Can you work these out from the model? Positions are in its coordinate system, mm. Face numbers are marked on the shaded views. A direction names the side the tool comes from. Round coordinates to 2 decimals unless told otherwise and drop trailing zeros. Loops run counter-clockwise (first coordinate to the right, second up) from the corner with the lowest first, then second, coordinate; pieces in that order, holes last.
(1) I want a section at C-C on x = 223. Write out the boundary of the cut face in (y, z).
(2) I want a section at A-A on y = -32. Write out the boundary of the cut face in (x, z).
(3) Thinking about a two-plate mould opening in Y: for the marked faces 3 and 4, which applies, released by +Y, released by -Y, zero draft, split by the parting line, or undercut?
(4) Which directions (+Z, -Z, +X, -X, +Y, -Y) give clear straight access to the entire face, cutting with the end or side of a thin tool? Please do the marked faces 1 and 2.
(5) If I drill on line 1 along Y through (x, z) = (129, 12); line 2 along Z through (x, y) = (30, -19); line 3 along Z through (x, y) = (85, -36), over which ranges is the centre line in solid material (lowest first)?
(6) I want a section at B-B on z = 59. Write out the boundary of the cut face in (x, y), plus the area to 3 significant figures.
(7) Will these pins go through, and if not, where does the flat tip stop? pin 1 Ø5 at (y, z) = (-23, 15.5) entering from -X; pin 2 Ø12 at (x, y) = (137.5, -37) entering from +Z; pin 3 Ø1 at (y, z) = (7.5, 10) entering from -X; pin 4 Ø5 at (y, z) = (-42.5, 15.5) entering from -X.
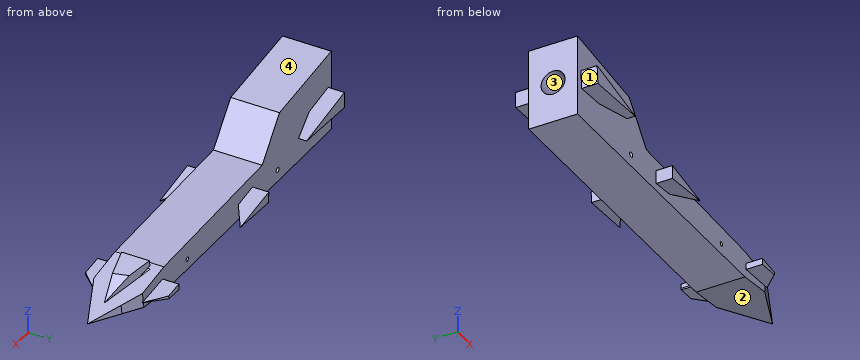
from build123d import *

# Parameters (mm, degrees)
F1_DEPTH  = 38.1
F4_DEPTH  = 38.1
F6_DEPTH  = 38.1
F8_DEPTH  = 38.1
F11_DEPTH = 12.7
F13_DEPTH = 12.7
F15_DEPTH = 12.7
F17_DEPTH = 25.4
F19_DEPTH = 7.62
F21_DEPTH = 25.4
F23_DEPTH = 12.7
F25_DEPTH = 12.7
F26_DEPTH = 12.7
F28_DEPTH = 25.4
F30_DEPTH = 25.4
F32_DEPTH = 25.4
F34_DEPTH = 25.4
F36_DEPTH = 25.4
F38_DEPTH = 25.4
F2_R      = 9.3756609964
F39_DEPTH = 50.8
F41_DEPTH = 25.4
F43_DEPTH = 25.4
F44_R     = 1.6440489173
F44_R_2   = 2.0037736154
F45_DEPTH = 50.8


with BuildPart() as f1:
    # F0 (on Front) → F1 (new body)
    with BuildSketch(Plane.XZ):
        Polygon((0, 63.5), (0, 0), (302.4093748547, 0), (302.4093748547, 25.4), align=None)
    extrude(amount=F1_DEPTH)

    # F3 (on face) → F4 (cut)
    with BuildSketch(Plane.XZ.offset(38.1)):
        Polygon((302.4093748547, 25.4), (71.378469884, 54.507158082), (95.2177494764, 25.4), (302.4093748547, 18.0674288422), align=None)
    extrude(amount=-F4_DEPTH, mode=Mode.SUBTRACT)

    # F5 (on face) → F6 (cut)
    with BuildSketch(Plane.XZ.offset(38.1)):
        Polygon((230.7509960012, 20.6034394606), (302.4093748547, 9.0337144211), (302.4093748547, 18.0674288422), align=None)
    extrude(amount=-F6_DEPTH, mode=Mode.SUBTRACT)

    # F7 (on face) → F8 (cut)
    with BuildSketch(Plane.XZ.offset(38.1)):
        Polygon((302.4093748547, 0), (302.4093748547, 9.0337144211), (230.7509960012, 0), align=None)
    extrude(amount=-F8_DEPTH, mode=Mode.SUBTRACT)

    # F10 (on face) → F11 (join)
    with BuildSketch(Plane.XZ.offset(38.1)):
        Polygon((57.0245832205, 26.8944967538), (4.6469587833, 37.9372723401), (5.7158898562, 24.0447483957), align=None)
    extrude(amount=F11_DEPTH)

    # F12 (on face) → F13 (join)
    with BuildSketch(Plane.XZ.offset(38.1)):
        Polygon((146.5801596642, 9.3731330708), (108.4925159812, 16.2170082331), (108.4925159812, 5.8024153113), align=None)
    extrude(amount=F13_DEPTH)

    # F14 (on face) → F15 (join)
    with BuildSketch(Plane.XZ.offset(38.1)):
        Polygon((261.0786855221, 8.5403770208), (232.2574704885, 11.8147395551), (232.5303256512, 7.1419519372), align=None)
    extrude(amount=F15_DEPTH)

    # F16 (on face) → F17 (cut)
    with BuildSketch(Plane(origin=(6.216250911, 0, 34.5947791457), x_dir=(0.9842368971, 0, -0.1768551111), z_dir=(0.1768551111, 0, 0.9842368971))):
        Polygon((123.2630957695, -38.1), (142.6119150394, -50.8), (142.6119150394, -38.1), align=None)
    extrude(amount=-F17_DEPTH, mode=Mode.SUBTRACT)

    # F18 (on face) → F19 (join)
    with BuildSketch(Plane(origin=(9.1045026508, 0, 56.3897497994), x_dir=(0.9872152882, 0, -0.159392518), z_dir=(0.159392518, 0, 0.9872152882))):
        Polygon((273.6749947071, -19.05), (230.3751856089, -7.3024798185), (230.3751856089, -29.0318094194), align=None)
    extrude(amount=F19_DEPTH)

    # F20 (on face) → F21 (cut)
    with BuildSketch(Plane(origin=(17.7501025045, -77.9948093822, -2.8658728914), x_dir=(0.9751003181, 0.2216146645, 0.0081430991), z_dir=(0.2217642207, -0.9744427175, -0.0358053182))):
        Polygon((238.2592436798, 18.4212918256), (225.1080880547, 25.1705576425), (224.3710737528, 20.7224409643), align=None)
    extrude(amount=-F21_DEPTH, mode=Mode.SUBTRACT)

    # F22 (on face) → F23 (join)
    with BuildSketch(Plane.XZ):
        Polygon((56.3897466524, 26.9276275739), (4.3465946801, 36.552254676), (4.3465946801, 24.2511220276), align=None)
    extrude(amount=-F23_DEPTH)

    # F24 (on face) → F25 (join)
    with BuildSketch(Plane.XZ):
        Polygon((232.4568778276, 11.635161005), (232.4568778276, 8.2633461603), (232.5210973665, 7.0146331797), (260.5405604993, 8.4556344572), align=None)
    extrude(amount=-F25_DEPTH)

    # F9 (on Front) → F26 (join)
    with BuildSketch(Plane.XZ):
        Polygon((147.8346826, 9.0159667453), (108.4925159812, 15.3243280947), (108.9198718135, 7.0146331797), align=None)
    extrude(amount=-F26_DEPTH)

    # F27 (on face) → F28 (cut)
    with BuildSketch(Plane(origin=(5.115117276, 0, 31.900486513), x_dir=(0.9873872694, 0, -0.1583236568), z_dir=(0.1583236568, 0, 0.9873872694))):
        Polygon((144.5426427436, 12.7), (124.6202840907, 0), (144.5426427436, 0), align=None)
    extrude(amount=-F28_DEPTH, mode=Mode.SUBTRACT)

    # F29 (on face) → F30 (cut)
    with BuildSketch(Plane(origin=(4.2425164902, 0, 37.4727133277), x_dir=(0.9936520123, 0, -0.1124974594), z_dir=(0.1124974594, 0, 0.9936520123))):
        Polygon((257.9354148407, 12.7), (243.803866611, 12.7), (257.9354148407, 0), align=None)
    extrude(amount=-F30_DEPTH, mode=Mode.SUBTRACT)

    # F31 (on face) → F32 (cut)
    with BuildSketch(Plane(origin=(4.2847349057, 0, 37.7145978145), x_dir=(0.993608254, 0, -0.1128832923), z_dir=(0.1128832923, 0, 0.993608254))):
        Polygon((258.4458709906, -50.8), (258.4458709906, -38.1), (246.229827404, -50.8), align=None)
    extrude(amount=-F32_DEPTH, mode=Mode.SUBTRACT)

    # F33 (on face) → F34 (cut)
    with BuildSketch(Plane(origin=(17.7501025045, -77.9948093822, -2.8658728914), x_dir=(0.9751003181, 0.2216146645, 0.0081430991), z_dir=(0.2217642207, -0.9744427175, -0.0358053182))):
        Polygon((269.454439727, 20.9764088194), (247.5355495769, 24.6081785526), (268.208854053, 13.4589014978), align=None)
    extrude(amount=-F34_DEPTH, mode=Mode.SUBTRACT)

    # F35 (on face) → F36 (cut)
    with BuildSketch(Plane(origin=(7.8556900223, 0, 37.2607754701), x_dir=(0.9784898364, 0, -0.2062950314), z_dir=(0.2062950314, 0, 0.9784898364))):
        Polygon((23.4852526042, -38.1), (50.2497740567, -44.45), (50.2497740567, -38.1), align=None)
    extrude(amount=-F36_DEPTH, mode=Mode.SUBTRACT)

    # F37 (on face) → F38 (cut)
    with BuildSketch(Plane(origin=(6.6800047408, 0, 36.1207242852), x_dir=(0.9833259332, 0, -0.1818518877), z_dir=(0.1818518877, 0, 0.9833259332))):
        Polygon((50.552660346, 0), (50.552660346, 6.35), (24.0898415521, 0), align=None)
    extrude(amount=-F38_DEPTH, mode=Mode.SUBTRACT)

    # F2 (on face) → F39 (cut)
    with BuildSketch(Plane(origin=(0, 0, 0), x_dir=(0, -1, 0), z_dir=(-1, 0, 0))):
        with Locations((19.05, 31.75)):
            Circle(F2_R)
    extrude(amount=-F39_DEPTH, mode=Mode.SUBTRACT)

    # F40 (on face) → F41 (cut)
    with BuildSketch(Plane(origin=(9.1045026508, 0, 56.3897497994), x_dir=(0.9872152882, 0, -0.159392518), z_dir=(0.159392518, 0, 0.9872152882))):
        Polygon((269.2834402546, 0), (254.3958723545, 0), (270.9897734825, -7.4018547064), align=None)
        Polygon((269.2834402546, 0), (270.9897734825, -7.4018547064), (297.1032516572, -19.05), (297.1032516572, 0), align=None)
    extrude(amount=-F41_DEPTH, mode=Mode.SUBTRACT)

    # F42 (on face) → F43 (cut)
    with BuildSketch(Plane(origin=(9.1045026508, 0, 56.3897497994), x_dir=(0.9872152882, 0, -0.159392518), z_dir=(0.159392518, 0, 0.9872152882))):
        Polygon((297.1032516572, -38.1), (297.1032516572, -19.05), (254.0944516659, -38.1), align=None)
    extrude(amount=-F43_DEPTH, mode=Mode.SUBTRACT)

    # F44 (on face) → F45 (cut)
    with BuildSketch(Plane.XZ.offset(38.1)):
        with Locations((198.3555555344, 8.1828935072)):
            Circle(F44_R)
        with Locations((73.9755779505, 9.3731330708)):
            Circle(F44_R_2)
    extrude(amount=-F45_DEPTH, mode=Mode.SUBTRACT)


solid = f1.part
Filled sheet:
1. outline: (-38.1, 0) - (0, 0) - (0, 20.88) - (-38.1, 20.88) - close
2. outline: (0, 0) - (230.75, 0) - (272.18, 5.22) - (273.55, 13.69) - (230.75, 20.6) - (95.22, 25.4) - (71.38, 54.51) - (0, 63.5) - close; hole circle Ø4.01 at (73.98, 9.37); hole circle Ø3.29 at (198.36, 8.18)
3. face 3: undercut
3. face 4: zero draft
4. face 1: -Z, -X, -Y
4. face 2: -Z, +X, +Y, -Y
5. line 1: y = -50.8 to -39.14, -38.1 to 0, 0.54 to 12.7
5. line 2: z = 0 to 22.37, 41.13 to 59.72
5. line 3: z = 0 to 37.88
6. outline: (0, -38.1) - (35.72, -38.1) - (35.72, 0) - (0, 0) - close
6. area: 1,360 mm2
7. pin 1: stops at x = 0
7. pin 2: stops at z = 24.12
7. pin 3: stops at x = 108.74
7. pin 4: stops at x = 108.49
